The listing builds one solid part. Answer for the finished solid, in the listing's coordinates (mm). A direction names the side the tool comes from. Round coordinates to 2 decimals unless told otherwise and drop trailing zeros. Write each loop counter-clockwise with the first axis right and the second up, starting at its lowest first coordinate (ties: lowest second). Pieces come first, ordered by that corner, then holes. Notation, with made-up numbers: (38, -20.5) - (70, -20.5) arc R7 ccw to (70, -9.5) - close; hole circle Ø7 at (24, -27). An arc over 180 degrees is marked (long way). Use a Markdown table: item, result. Add a question column.
1) Find the intervals of material crossed by probe 1 along X at (y, z) = (-4, 2.25); probe 2 along Z at (x, y) = (21, -3.75); probe 3 along X at (y, z) = (-3, -0.5), in increasing order. Write a range as from..to.
2) A cutting plane is placed at B-B (y = -1.5). Give the vertices of the cut face in (x, z).
3) A cutting plane is placed at A-A (z = 11). Give the vertices of the cut face in (x, y).
4) Each of these flat-tipped pins is pushed along its axis until it touches: P1, Ø2, axis at x = 83, y = -1, coming from the -Z side; P2, Ø1.3, axis at x = -1.5, y = -4, coming from the -Z side; P3, Ø1, axis at x = 25, y = -4.5, coming from the +Z side. Where does it stop, or does it pass through?
5) A tool of negligible diameter and unlimited length cuts with its end or side. For faces 4 (the flat face through (1.409, -3, 2)), 5 (the flat face through (97.7, -4.1, -0.3)), 6 (the flat face through (95.409, -3, 11)), from which of +Z, -Z, +X, -X, +Y, -Y can it reach the whole face along a straight path? Write none if from no direction.
6) A cutting plane is placed at C-C (x = 87.5). Give the vertices of the cut face in (y, z), then the cut area to 3 significant figures.
7) Determine the mould class of faces 1 (the flat face through (48, -3, 9.5)), 2 (the flat face through (101.409, -3, 7)), 3 (the flat face through (48, -0.427, 7)) for opening direction X: +X half, -X half, draft (parallel to the pull), parting line (faces both ways), or undercut.
```python
from build123d import *

# Parameters (mm, degrees)
SKETCH_1_W      = 6
SKETCH_1_H      = 6
EXTRUDE_1_DEPTH = 13
SKETCH_3_R      = 0.8
EXTRUDE_3_DEPTH = 1.6
SKETCH_4_W      = 6
SKETCH_4_H      = 3
EXTRUDE_4_DEPTH = 94
SKETCH_5_W      = 13.6
SKETCH_5_H      = 6
EXTRUDE_5_DEPTH = 6
SKETCH_2_R      = 0.8
EXTRUDE_2_DEPTH = 1.6
SKETCH_7_R      = 0.8
EXTRUDE_6_DEPTH = 1.6


with BuildPart() as part:
    # 草图1 → 凸台-拉伸1 (new body)
    with BuildSketch(Plane.XY):
        with Locations((-1.59089175, -3.42724845)):
            Rectangle(SKETCH_1_W, SKETCH_1_H)
    extrude(amount=EXTRUDE_1_DEPTH)

    # 草图3 → 凸台-拉伸3 (add)
    with BuildSketch(Plane(origin=(0, 0, 0), x_dir=(-1, 0, 0), z_dir=(0, 0, -1))):
        with Locations((1.59089175, -3.42724845)):
            Circle(SKETCH_3_R)
    extrude(amount=EXTRUDE_3_DEPTH)

    # 草图4 → 凸台-拉伸4 (add)
    with BuildSketch(Plane(origin=(1.40910825, 0, 0), x_dir=(0, 0, -1), z_dir=(1, 0, 0))):
        with Locations((-6.5, -4.92724845)):
            Rectangle(SKETCH_4_W, SKETCH_4_H)
        with Locations((-6.5, -1.92724845)):
            Rectangle(SKETCH_4_W, SKETCH_4_H)
    extrude(amount=EXTRUDE_4_DEPTH)

    # 草图5 → 凸台-拉伸5 (add)
    with BuildSketch(Plane(origin=(95.40910825, 0, 0), x_dir=(0, 0, -1), z_dir=(1, 0, 0))):
        with Locations((-6.5, -3.42724845)):
            Rectangle(SKETCH_5_W, SKETCH_5_H)
    extrude(amount=EXTRUDE_5_DEPTH)

    # 草图2 → 凸台-拉伸2 (add)
    with BuildSketch(Plane.XY.offset(13)):
        with Locations((-1.59089175, -3.42724845)):
            Circle(SKETCH_2_R)
        with Locations((98.40910825, -3.42724845)):
            Circle(SKETCH_2_R)
    extrude(amount=EXTRUDE_2_DEPTH)

    # 草图7 → 凸台-拉伸6 (add)
    with BuildSketch(Plane(origin=(0, 0, -0.3), x_dir=(-1, 0, 0), z_dir=(0, 0, -1))):
        with Locations((-98.40910825, -3.42724845)):
            Circle(SKETCH_7_R)
    extrude(amount=EXTRUDE_6_DEPTH)


solid = part.part
```
Entries:
| question | item | result |
|---|---|---|
| 1 | probe 1 | x = -4.59..1.41, 95.41..101.41 |
| 1 | probe 2 | z = 3.5..9.5 |
| 1 | probe 3 | x = -2.27..-0.91, 97.73..99.09 |
| 2 | outline | (-4.59, 0) - (1.41, 0) - (1.41, 3.5) - (95.41, 3.5) - (95.41, -0.3) - (101.41, -0.3) - (101.41, 13.3) - (95.41, 13.3) - (95.41, 9.5) - (1.41, 9.5) - (1.41, 13) - (-4.59, 13) - close |
| 3 | outline | (-4.59, -6.43) - (1.41, -6.43) - (1.41, -0.43) - (-4.59, -0.43) - close; (95.41, -6.43) - (101.41, -6.43) - (101.41, -0.43) - (95.41, -0.43) - close |
| 4 | P1 | stops at z = 3.5 |
| 4 | P2 | stops at z = -1.6 |
| 4 | P3 | stops at z = 9.5 |
| 5 | face 4 | -Z, +Y, -Y |
| 5 | face 5 | -Z |
| 5 | face 6 | +Z, +Y, -Y |
| 6 | outline | (-6.43, 3.5) - (-0.43, 3.5) - (-0.43, 9.5) - (-6.43, 9.5) - close |
| 6 | area | 36.0 mm² |
| 7 | face 1 | undercut |
| 7 | face 2 | +X half |
| 7 | face 3 | draft |
